```python
from build123d import *

# Parameters (mm, degrees)
SKETCH1_R           = 1.8
SKETCH1_R_2         = 1.2
SKETCH1_R_3         = 2
BOSS_EXTRUDE1_DEPTH = 7
SKETCH1_3_W         = 20
SKETCH1_3_H         = 6
SKETCH1_3_R         = 1.8
CUT_EXTRUDE1_DEPTH  = 5
FILLET1_R           = 3
CHAMFER3_SIZE       = 0.7
CUT_EXTRUDE2_DEPTH  = 29.072613197
FILLET2_R           = 10
FILLET3_R           = 3


with BuildPart() as part:
    # Sketch1 → Boss-Extrude1 (new, symmetric)
    with BuildSketch(Plane(origin=(0, 0, 0), x_dir=(1, 0, 0), z_dir=(0, 1, 0))):
        with BuildLine():
            Line((10, 5), (-10, 5))
            Line((-10, 5), (-10, -5))
            ThreePointArc((-10, -5), (-8.073014031, -10.781966564), (-4.004817267, -15.320048466))
            Line((-4.004817267, -15.320048466), (-3, -16))
            Line((-3, -16), (3, -16))
            Line((3, -16), (11.972113592, -10.011064555))
            Line((11.972113592, -10.011064555), (11.999968963, -5.011142148))
            Line((11.999968963, -5.011142148), (10, -5))
            Line((10, -5), (10, 5))
        make_face()
        with Locations(Location((-5, 2, 0), (0, 0, 270))):
            Circle(SKETCH1_R, mode=Mode.SUBTRACT)
        with Locations(Location((5, 2, 0), (0, 0, 270))):
            Circle(SKETCH1_R, mode=Mode.SUBTRACT)
        with Locations(Location((8.477738981, -8.991581315, 0), (0, 0, 270))):
            Circle(SKETCH1_R_2, mode=Mode.SUBTRACT)
        with Locations(Location((0, -12, 0), (0, 0, 270))):
            Circle(SKETCH1_R_3, mode=Mode.SUBTRACT)
    extrude(amount=BOSS_EXTRUDE1_DEPTH, both=True)

    # Sketch1<3> → Cut-Extrude1 (cut, symmetric)
    # profile 1 of 2: a face of its own
    with BuildSketch(Plane(origin=(0, 0, 0), x_dir=(1, 0, 0), z_dir=(0, 1, 0))):
        with Locations((0, 2)):
            Rectangle(SKETCH1_3_W, SKETCH1_3_H)
        with Locations(Location((-5, 2, 0), (0, 0, 270))):
            Circle(SKETCH1_3_R, mode=Mode.SUBTRACT)
        with Locations(Location((5, 2, 0), (0, 0, 270))):
            Circle(SKETCH1_3_R, mode=Mode.SUBTRACT)
    # profile 2 of 2: a face of its own
    with BuildSketch(Plane(origin=(0, 0, 0), x_dir=(1, 0, 0), z_dir=(0, 1, 0))):
        with BuildLine():
            Line((-3, -16), (-4.004817267, -15.320048466))
            ThreePointArc((-4.004817267, -15.320048466), (-3.509286078, -15.670187568), (-3, -16))
        make_face()
    extrude(amount=CUT_EXTRUDE1_DEPTH, both=True, mode=Mode.SUBTRACT)

    # Fillet1
    fillet1_edges = [part.edges().sort_by_distance(p)[0] for p in [
        (-10, 6, -5),
        (10, 6, -5),
        (-10, -6, -5),
        (10, -6, -5),
    ]]
    fillet(fillet1_edges, radius=FILLET1_R)

    # Chamfer3
    chamfer3_edges = [part.edges().sort_by_distance(p)[0] for p in [
        (10, -7, 1.5),
        (-10, 7, 1.5),
        (-10, -7, 1.5),
        (10, 7, 1.5),
        (0, -7, -5),
        (9.121320344, -7, -4.121320344),
        (-9.121320344, -7, -4.121320344),
        (0, 7, -5),
        (9.121320344, 7, -4.121320344),
        (-9.121320344, 7, -4.121320344),
    ]]
    chamfer(chamfer3_edges, length=CHAMFER3_SIZE)

    # Sketch2 → Cut-Extrude2 (cut, through all)
    with BuildSketch(Plane(origin=(12.027513532, 0, 0.067007209), x_dir=(0.005571074109334343, 0, -0.9999844814462214), z_dir=(0.9999844814462214, 0, 0.005571074109334343))):
        Polygon((-20.022955032, 1.5), (-20.022955032, 7), (-1.768785186, 7), (-4.944211666, 1.5), align=None)
        Polygon((-20.050357448, -7), (-20.050357448, -1.5), (-4.944211666, -1.5), (-1.768785186, -7), align=None)
    extrude(amount=-CUT_EXTRUDE2_DEPTH, mode=Mode.SUBTRACT)

    # Fillet2
    # the kernel refuses this fillet: 10 mm, written as the material it adds along each edge
    with BuildSketch(Plane(origin=(10, 16.472041172, 5), x_dir=(0, 0, -1), z_dir=(0, -1, 0))) as fillet2_piece_1_section:
        with BuildLine():
            CenterArc((5.988816469, 10), FILLET2_R, 233.130398738, 36.869601262)
            Line((-0.011142148, 1.999968963), (0, 0))
            Line((0, 0), (5.988816469, 0))
        make_face()
    fillet2_piece_1 = extrude(amount=32.944082344, mode=Mode.PRIVATE)
    fillet2_piece_1 = split(fillet2_piece_1, bisect_by=Plane(origin=(10, 5, 5), z_dir=(0, 1, 0)), keep=Keep.TOP, mode=Mode.PRIVATE)
    fillet2_piece_1 = split(fillet2_piece_1, bisect_by=Plane(origin=(10.036117741, 12.729030879, -1.482983393), z_dir=(0.004824691705049313, -0.4999999999999978, -0.8660119643226377)), keep=Keep.TOP, mode=Mode.PRIVATE)
    fillet2_piece_1 = split(fillet2_piece_1, bisect_by=Plane(origin=(4.913979414, 11.386020586, 5), z_dir=(-0.707106781186548, -0.7071067811865471, 0)), keep=Keep.TOP, mode=Mode.PRIVATE)
    add(fillet2_piece_1)
    with BuildSketch(Plane(origin=(10, 16.472041172, 5), x_dir=(0, 0, -1), z_dir=(0, -1, 0))) as fillet2_piece_2_section:
        with BuildLine():
            CenterArc((5.988816469, 10), FILLET2_R, 233.130398738, 36.869601262)
            Line((-0.011142148, 1.999968963), (0, 0))
            Line((0, 0), (5.988816469, 0))
        make_face()
    fillet2_piece_2 = extrude(amount=32.944082344, mode=Mode.PRIVATE)
    fillet2_piece_2 = split(fillet2_piece_2, bisect_by=Plane(origin=(10, 16.472041172, 1), z_dir=(0, 0, 1)), keep=Keep.TOP, mode=Mode.PRIVATE)
    fillet2_piece_2 = split(fillet2_piece_2, bisect_by=Plane(origin=(21.386020586, 5.086020586, 5), z_dir=(-0.707106781186548, 0.7071067811865471, 0)), keep=Keep.TOP, mode=Mode.PRIVATE)
    fillet2_piece_2 = split(fillet2_piece_2, bisect_by=Plane(origin=(9.956645221, 11.979030879, 12.782001339), z_dir=(0.004824691705049311, 0.4999999999999981, -0.8660119643226375)), keep=Keep.TOP, mode=Mode.PRIVATE)
    fillet2_piece_2 = split(fillet2_piece_2, bisect_by=Plane(origin=(10.036117741, 12.729030879, -1.482983393), z_dir=(0.004824691705049313, -0.4999999999999978, -0.8660119643226377)), keep=Keep.TOP, mode=Mode.PRIVATE)
    fillet2_piece_2 = split(fillet2_piece_2, bisect_by=Plane(origin=(4.913979414, 11.386020586, 5), z_dir=(-0.707106781186548, -0.7071067811865471, 0)), keep=Keep.TOP, mode=Mode.PRIVATE)
    add(fillet2_piece_2)
    with BuildSketch(Plane(origin=(10, 16.472041172, 5), x_dir=(0, 0, -1), z_dir=(0, -1, 0))) as fillet2_piece_3_section:
        with BuildLine():
            CenterArc((5.988816469, 10), FILLET2_R, 233.130398738, 36.869601262)
            Line((-0.011142148, 1.999968963), (0, 0))
            Line((0, 0), (5.988816469, 0))
        make_face()
    fillet2_piece_3 = extrude(amount=32.944082344, mode=Mode.PRIVATE)
    fillet2_piece_3 = split(fillet2_piece_3, bisect_by=Plane(origin=(10, -5, 5), z_dir=(0, -1, 0)), keep=Keep.TOP, mode=Mode.PRIVATE)
    fillet2_piece_3 = split(fillet2_piece_3, bisect_by=Plane(origin=(21.386020586, 5.086020586, 5), z_dir=(-0.707106781186548, 0.7071067811865471, 0)), keep=Keep.TOP, mode=Mode.PRIVATE)
    fillet2_piece_3 = split(fillet2_piece_3, bisect_by=Plane(origin=(9.956645221, 11.979030879, 12.782001339), z_dir=(0.004824691705049311, 0.4999999999999981, -0.8660119643226375)), keep=Keep.TOP, mode=Mode.PRIVATE)
    add(fillet2_piece_3)

    # Fillet3
    fillet3_edges = [part.edges().sort_by_distance(p)[0] for p in [
        (11.972113592, 0, 10.011064555),
        (3, 0, 16),
        (-3, 0, 16),
    ]]
    fillet(fillet3_edges, radius=FILLET3_R)


solid = part.part
```
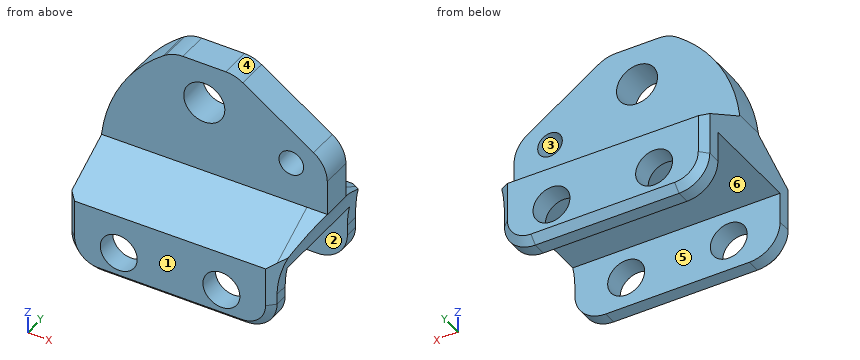
Read the model definition and answer for the solid it produces. Units are mm, in the model's axes. Face numbers are marked on the shaded views. A direction names the side the tool comes from. Coordinates: 2 decimals unless noted, no trailing zeros. Loops run counter-clockwise (first coordinate to the right, second up) from the corner with the lowest first, then second, coordinate; pieces in that order, holes last.
(1) A tool of negligible diameter and unlimited length cuts with its end or side. For the marked faces 1 and 2, from which of +Z, -Z, +X, -X, +Y, -Y can it reach the whole face along a straight path? Write none if from no direction.
Solution:
face 1: +Z, -Z, +X, -X, -Y
face 2: -Z, +X, -X
(2) The part is cut by section D-D (x = 5). Determine the outline of the cut face in (y, z).
Solution:
outline: (-7, -4.3) - (-6.3, -5) - (-5, -5) - (-5, -3.8) - (-7, -3.8) - close; (-7, -0.2) - (-5, -0.2) - (-5, 1) - (5, 1) - (5, -0.2) - (7, -0.2) - (7, 1.8) - (1.5, 4.97) - (1.5, 14.66) - (-1.5, 14.66) - (-1.5, 4.97) - (-7, 1.8) - close; (5, -5) - (6.3, -5) - (7, -4.3) - (7, -3.8) - (5, -3.8) - close
(3) The part is cut by section B-B (z = 9.25). Determine the outline of the cut face in (x, y).
Solution:
outline: (-8.85, -1.5) - (7.31, -1.5) - (7.31, 1.5) - (-8.85, 1.5) - close; (9.65, -1.5) - (11.86, -1.5) - (11.86, 1.5) - (9.65, 1.5) - close
(4) The part is cut by section C-C (x = 0). Determine the outline of the cut face in (y, z).
Solution:
outline: (-7, -4.3) - (-6.3, -5) - (-5, -5) - (-5, 1) - (5, 1) - (5, -5) - (6.3, -5) - (7, -4.3) - (7, 1.77) - (1.5, 4.94) - (1.5, 10) - (-1.5, 10) - (-1.5, 4.94) - (-7, 1.77) - close; (-1.5, 14) - (1.5, 14) - (1.5, 16) - (-1.5, 16) - close
(5) The mould has two halves that part along Z. Classify the marked faces 3, 4, 5 and 6: released by +Z, released by -Z, zero draft, split by the parting line, or undercut.
Solution:
face 3: undercut
face 4: released by +Z
face 5: zero draft
face 6: released by -Z
(6) Consider line 1 along X through (y, z) = (5.8, -2); line 2 along X through (y, z) = (6.4, -2); line 3 along Y through (x, z) = (6, 5). Determine where each line is inside the solid, lowest interval first.
Solution:
line 1: x = -10 to -6.8, -3.2 to 3.2, 6.8 to 10
line 2: x = -9.9 to -6.8, -3.2 to 3.2, 6.8 to 9.9
line 3: y = -1.5 to 1.5
(7) The part is cut by section A-A (y = 0). Determine the outline of the cut face in (x, z), and give its area (3 significant figures).
Solution:
outline: (-10, 1) - (10.2, 1) arc R10 cw to (12, 5.01) - (11.98, 8.42) arc R3 ccw to (10.65, 10.9) - (3.76, 15.5) arc R3 ccw to (2.09, 16) - (-2.08, 16) arc R3 ccw to (-3.76, 15.48) - (-4, 15.32) arc R15 ccw to (-10, 5) - close; hole circle Ø4 at (0, 12); hole circle Ø2.4 at (8.48, 8.99)
area: 256 mm2
(8) Flat-ended cylindrical pins translate along their axes: pin 1 Ø3 at (y, z) = (-2, 5.5) entering from -X; pin 2 Ø5.5 at (x, z) = (-3, 9.5) entering from -Y; pin 3 Ø0.5 at (y, z) = (6, -1.5) entering from +X; pin 4 Ø9 at (x, z) = (-2.5, 10.5) entering from +Y. Find the tip coordinate at first contact, or state that the pin passes through.
Solution:
pin 1: stops at x = -10
pin 2: stops at y = -1.5
pin 3: stops at x = 10
pin 4: stops at y = 1.5
